Autodesk Fusion 360 part; units mm, degrees
sketch "Szkic1" plane through (0, 0, 0) normal (0, 0, 1) x (1, 0, 0)
  line L0 (-25, 50.8) -> (345, 50.8)
  line L1 (345, 50.8) -> (345, -179.1)
  line L2 (345, -179.1) -> (-25, -179.1)
  line L3 (-25, -179.1) -> (-25, 50.8)
  line L4 (-20, 45.8) -> (340, 45.8)
  line L5 (340, 45.8) -> (340, -162.2)
  line L6 (340, -162.2) -> (-20, -162.2)
  line L7 (-20, -162.2) -> (-20, 45.8)
  line L8 (-10, -50) -> (330, -50)
  line L9 (330, -50) -> (330, -160)
  line L10 (330, -160) -> (-10, -160)
  line L11 (-10, -160) -> (-10, -50)
  dimension "d1" = 370
  dimension "d2" = 229.9
  dimension "d3" = 360
  dimension "d4" = 208
  dimension "d5" = 5
  dimension "d6" = 16.9
extrude "Wyciągnięcie proste1" add sketch "Szkic1" along normal blind 35 contours L0 L1 L2 L3
extrude "Wyciągnięcie proste2" add sketch "Szkic1" along normal blind 5 contours L4 L5 L6 L7 | L8 L9 L10 L11
sketch "Szkic2" plane through (-25, 0, 0) normal (-1, 0, 0) x (0, -1, 0)
  line L0 (-50.8, 0) -> (179.1, 0)
  line L1 (179.1, 0) -> (179.1, 35)
  line L2 (179.1, 35) -> (-50.8, 35)
  line L3 (-50.8, 35) -> (-50.8, 0)
  line L4 (-22.9208, 21.9096) -> (-8.9208, 21.9096)
  line L5 (-8.9208, 21.9096) -> (-8.9208, 14.9096)
  line L6 (-8.9208, 14.9096) -> (-22.9208, 14.9096)
  line L7 (-22.9208, 14.9096) -> (-22.9208, 21.9096)
  line L8 (-38.9208, 21.9096) -> (-8.9208, 21.9096)
  line L9 (-8.9208, 21.9096) -> (-8.9208, 14.9096)
  line L10 (-8.9208, 14.9096) -> (-38.9208, 14.9096)
  line L11 (-38.9208, 14.9096) -> (-38.9208, 21.9096)
  line L12 (-1.4208, 21.9096) -> (12.5792, 21.9096)
  line L13 (12.5792, 21.9096) -> (12.5792, 14.9096)
  line L14 (12.5792, 14.9096) -> (-1.4208, 14.9096)
  line L15 (-1.4208, 14.9096) -> (-1.4208, 21.9096)
  circle A0 centre (24.0792, 18.4096) radius 3.25
  dimension "d11" = 14
  dimension "d12" = 7
  dimension "d13" = 30
  dimension "d14" = 7
  dimension "d15" = 14
  dimension "d16" = 7
  dimension "d17" = 7.5
  dimension "d18" = 6.5
  dimension "d19" = 11.5
extrude "Wyciągnięcie proste3" cut sketch "Szkic2" against normal blind 3 contours L4 L5 L6 L7 L8 L9 L10 | L12 L13 L14 L15 | A0
extrude "Wyciągnięcie proste4" cut 3 faces at (-22, 18.2542, 17.2429) (-22, -3.2458, 19.5763) (-22, -23.249, 17.192) along direction (1, 0, 0) blind 2
sketch "Szkic3" plane through (345, 0, 0) normal (1, 0, 0) x (0, 1, 0)
  line L0 (-179.1, 0) -> (50.8, 0)
  line L1 (50.8, 0) -> (50.8, 35)
  line L2 (50.8, 35) -> (-179.1, 35)
  line L3 (-179.1, 35) -> (-179.1, 0)
  line L4 (-50, 20.91) -> (0, 20.91)
  line L5 (0, 20.91) -> (0, 14.91)
  line L6 (0, 14.91) -> (-50, 14.91)
  line L7 (-50, 14.91) -> (-50, 20.91)
  line L8 (50.8, 0) -> (-179.1, 0)
  dimension "d24" = 50
  dimension "d25" = 6
  dimension "d26" = 14.91
extrude "Wyciągnięcie proste5" cut sketch "Szkic3" against normal blind 50 contours L4 L5 L6 L7
extrude "Wyciągnięcie proste6" cut sketch "Szkic2" against normal blind 450 contours L7 L8 L10 L11
sketch "Szkic4" plane through (0, -179.1, 0) normal (0, -1, 0) x (1, 0, 0)
  line L0 (-25, 0) -> (345, 0)
  line L1 (345, 0) -> (345, 35)
  line L2 (345, 35) -> (-25, 35)
  line L3 (-25, 35) -> (-25, 0)
  line L4 (0, 0) -> (320, 0)
  line L5 (320, 0) -> (320, 24.5591)
  line L6 (320, 24.5591) -> (0, 24.5591)
  line L7 (0, 24.5591) -> (0, 0)
  dimension "d31" = 320
  dimension "d32" = 25
extrude "Wyciągnięcie proste7" cut sketch "Szkic4" against normal blind 100 contours L0 L4 L5 L6 L7
extrude "Wyciągnięcie proste8" cut sketch "Szkic4" against normal blind 120 contours L0 L4 L5 L6 L7
extrude "Wyciągnięcie proste9" add sketch "Szkic1" along normal blind 5 contours L8 L9 L10 L11
extrude "Wyciągnięcie proste10" cut sketch "Szkic4" against normal blind 100 contours L0 L4 L5 L6 L7
sketch "Szkic5" plane through (0, 50.8, 0) normal (0, 1, 0) x (-1, 0, 0)
  line L0 (-345, 0) -> (25, 0)
  line L1 (25, 0) -> (25, 35)
  line L2 (25, 35) -> (-345, 35)
  line L3 (-345, 35) -> (-345, 0)
  line L4 (-345, 25.3824) -> (25, 25.3824)
  line L5 (25, 25.3824) -> (25, 0)
  line L6 (25, 0) -> (-345, 0)
  line L7 (-345, 0) -> (-345, 25.3824)
  line L8 (-340, 25.3824) -> (20, 25.3824)
  line L9 (20, 25.3824) -> (20, 0)
  line L10 (20, 0) -> (-340, 0)
  line L11 (-340, 0) -> (-340, 25.3824)
  dimension "d41" = 360
  dimension "d42" = 5
extrude "Wyciągnięcie proste11" add sketch "Szkic5" along normal blind 15 contours L0 L4 L6 L8 L9 L10 L11
extrude "Wyciągnięcie proste12" cut 1 faces at (220, 65.8, 16.9216) along direction (0, -1, 0) blind 18
extrude "Wyciągnięcie proste13" cut 1 faces at (220, 47.8, 16.9216) along direction (0, -1, 0) blind 20
extrude "Wyciągnięcie proste14" add sketch "Szkic5" along normal blind 35 contours L0 L3 L4 L6 L7 L11 | L1 L2 L3 L4 L8 | L0 L1 L4 L5 L6 L9
equation "d22 = 0 mm - 2.00 mm"
Source: CAD feature listing. Evaluate the final solid. Frame: model axes, mm. A direction names the side the tool comes from. Round coordinates to 2 decimals unless told otherwise and drop trailing zeros. Order: outer loops, then holes, each group sorted by start corner. A loop starts at its lowest first (then second) coordinate and runs counter-clockwise, first axis right, second up. Notation, with made-up numbers: (-19.75, 26.25) - (2.25, 26.25) arc R25 cw to (2.25, 53.25) - close; hole circle Ø1 at (81.25, -20). An arc over 180 degrees is marked (long way). Use a Markdown table: item, result. Add a question column.
1. Section query D-D (y = -154). Return the cut outline in (x, z), then the cut area to 3 significant figures.
2. First-contact query: pin 1 (1.5 mm diameter, centred on x = 95.5, z = 2.5, fed in from -Y); pin 2 (3 mm diameter, centred on x = 193.5, y = 1, fed in from +Z); pin 3 (2.5 mm diameter, centred on x = 131.5, z = 3.5, fed in from +Y); pin 4 (6 mm diameter, centred on x = 135.5, z = 10, fed in from +Y) (1 decimal). Flat tips, straight axial feed; report the tip coordinate or a pass-through.
3. Section query A-A (x = 190). Return the cut outline in (y, z), then the cut area to 3 significant figures.
4. Mould query, pull axis X, two halves, no side actions, for faces 4 (the flat face through (163, 66, 25.382)), 5 (the flat face through (345, -44.8, 21.1)), 6 (the flat face through (161, 85.8, 32)). Classes: +X half, -X half, draft (parallel to the pull), parting line (faces both ways), or undercut.
5. Section query C-C (z = 10.5). Return the cut outline in (x, y).
6. Line query: probe 1 along X at (y, z) = (-70.5, 19.5); probe 2 along Y at (x, z) = (178.5, 27); probe 3 along Y at (x, z) = (140.5, 25). Output: solid intervals per line, ascending.
7. Section query B-B (y = -5.5). Return the cut outline in (x, z).
8. Set-up query: faces 1 (the flat face through (162, -171, 24.559)), 2 (the flat face through (320, -152, 4)), 3 (the flat face through (-20, -36, 18)). Return all of +Z, -Z, +X, -X, +Y, -Y with unobstructed straight access to the full face (end or side cutting, diameter ignored); none if empty.
Derived:
| question | item | result |
|---|---|---|
| 1 | outline | (-25, 0) - (0, 0) - (0, 5) - (-20, 5) - (-20, 35) - (-25, 35) - close; (320, 0) - (345, 0) - (345, 35) - (340, 35) - (340, 5) - (320, 5) - close |
| 1 | area | 550 mm2 |
| 2 | pin 1 | y = -79.1 |
| 2 | pin 2 | z = 5 |
| 2 | pin 3 | y = 27.8 |
| 2 | pin 4 | through |
| 3 | outline | (-179.1, 24.56) - (-162.2, 24.56) - (-162.2, 35) - (-179.1, 35) - close; (-79.1, 0) - (27.8, 0) - (27.8, 5) - (-79.1, 5) - close; (45.8, 25.38) - (85.8, 25.38) - (85.8, 35) - (45.8, 35) - close |
| 3 | area | 1,100 mm2 |
| 4 | face 4 | undercut |
| 4 | face 5 | +X half |
| 4 | face 6 | draft |
| 5 | outline | (-25, -179.1) - (0, -179.1) - (0, -162.2) - (-20, -162.2) - (-20, 85.8) - (-25, 85.8) - close; (320, -179.1) - (345, -179.1) - (345, 85.8) - (340, 85.8) - (340, -162.2) - (320, -162.2) - close |
| 6 | probe 1 | -25 to -20, 340 to 345 |
| 6 | probe 2 | -179.1 to -162.2, 45.8 to 85.8 |
| 6 | probe 3 | -179.1 to -162.2 |
| 7 | outline | (-25, 0) - (345, 0) - (345, 14.91) - (340, 14.91) - (340, 5) - (-20, 5) - (-20, 14.91) - (-25, 14.91) - close; (-25, 21.91) - (-20, 21.91) - (-20, 35) - (-25, 35) - close; (340, 20.91) - (345, 20.91) - (345, 35) - (340, 35) - close |
| 8 | face 1 | -Z, +Y, -Y |
| 8 | face 2 | -Z, -Y |
| 8 | face 3 | none |
